Check sheet for the modelled part. Datum: model origin and axes. Units: mm. A direction names the side the tool comes from. Give positions to 0.01 mm unless a question says otherwise; leave off trailing zeros. Loops run counter-clockwise (first coordinate to the right, second up) from the corner with the lowest first, then second, coordinate; pieces in that order, holes last. Notation, with made-up numbers: (65.25, -22) -> (123.25, -22) arc R20 ccw to (123.25, 8) -> close; hole circle Ø2 at (43, -3.75). An arc over 180 degrees is marked (long way). Write each question's results on one line, items separated by ' | '. Start each with the question number.
Item 1: Scan lines: line 1 along X through (y, z) = (-4.75, 5.2); line 2 along Z through (x, y) = (3.7, -4.8); line 3 along Z through (x, y) = (15.5, 11.5). Record each from-to range of solid material in increasing order.
Item 2: Cross-section at A-A on x = 12.7. Enter the section's corners in (y, z).
Item 3: Access from +Z, -Z, +X, -X, +Y, -Y to the whole of each face (thin tool, end or side, straight path). Record for faces 4 (the face through (6, -5.427, 3)), 5 (the face through (-1.3, -4, 5)), 6 (the face through (8, -3.427, 7)).
Item 4: Cross-section at D-D on z = 0.75. Enter the section's corners in (x, y).
Item 5: Gauge pin test, flat ends, axial feed: pin 1 Ø2 at (x, z) = (12.7, 5.2) entering from +Y (1 decimal); pin 2 Ø4 at (y, z) = (1.5, 3) entering from -X; pin 3 Ø5 at (y, z) = (2.5, 2) entering from +X; pin 4 Ø5 at (x, z) = (-15, 1) entering from +Y. Record the tip position at first contact, or that the pin passes through.
Item 6: Mould release check, pull along X, two halves, no side actions. Record for faces 1 (the face through (0, 5, 2)), 2 (the face through (-18.003, -15.713, 0.986)), 3 (the face through (-12.435, -12.035, 0.986)): pulls with the +X half, pulls with the -X half, needs draft (parallel to the pull), parting line crosses it, or undercut.
Item 7: Cross-section at B-B on z = 5.2. Enter the section's corners in (x, y).
Autodesk Inventor part; units mm, degrees
ref_plane "Work Plane2" through (-1.3, -10.427, 8.7) normal (0, 0, 1) x (1, 0, 0)
ref_plane "YZ Plane" through (0, 0, 0) normal (1, 0, 0) x (0, 1, 0)
ref_plane "XZ Plane" through (0, 0, 0) normal (0, 1, 0) x (-1, 0, 0)
ref_plane "Work Plane1" through (0, 0, 0) normal (0, 0, 1) x (1, 0, 0)
sketch "Sketch2" plane through (0, 0, 0) normal (0, 0, 1) x (1, 0, 0)
  circle A0 centre (-17.6777, 17.6777) radius 3
  circle A1 centre (17.6777, 17.6777) radius 3
  circle A2 centre (-17.6777, -17.1777) radius 3
  line L0 (17.7, -5.427) -> (-1.3, -5.427)
  line L1 (-1.3, -5.427) -> (17.7, -5.427)
  line L2 (17.7, -5.427) -> (17.7, -3.927)
  line L3 (17.7, -3.927) -> (-1.3, -3.927)
  line L4 (-1.3, -3.927) -> (-1.3, -5.427)
  arc A3 (-15.9573, 20.1354) -> (15.9573, 20.1354) centre (0, 42.9323) ccw
  arc A4 (-20.3689, -15.8521) -> (-20.3689, 16.3521) centre (-53.0613, 0.25) ccw
  arc A5 (-14.9864, -18.5032) -> (-11, -5.427) centre (-53.0613, 0.25) ccw
  line L5 (-11, -5.427) -> (-1.3, -5.427)
  arc A6 (20.5658, 16.8661) -> (17.7, -3.927) centre (94.5659, -3.927) ccw
  circle A7 centre (-17.6777, 17.6777) radius 1.5
  circle A8 centre (17.6777, 17.6777) radius 1.5
  circle A9 centre (-17.6777, -17.1777) radius 1.5
  point P0 (0, 0)
  point P1 (-10.5, -5.427)
  dimension "d6" = 19
  dimension "d7" = 1.5
  dimension "d9" = 0.5
  dimension "d10" = 3
  dimension "d11" = 3
  dimension "d12" = 3
extrude "Extrusion1" add sketch "Sketch2" along normal blind 2
sketch "Sketch3" plane through (0, 0, 2) normal (0, 0, 1) x (1, 0, 0)
  line L0 (-11, -5.427) -> (17.7, -5.427)
  line L1 (17.7, -5.427) -> (-1.3, -5.427)
  line L2 (-1.3, -5.427) -> (-1.3, -3.427)
  line L3 (-1.3, -3.427) -> (17.7, -3.427)
  line L4 (17.7, -3.427) -> (17.7, -5.427)
  point P0 (0, 0)
  dimension "d15" = 19
  dimension "d16" = 2
ref_plane "Work Plane2" through (-1.3, -10.427, 8.7) normal (0, 0, 1) x (1, 0, 0)
extrude "Extrusion2" add sketch "Sketch3" along normal up to surface (6.7 mm away)
sketch "Sketch4" plane through (-1.3, -3.427, 2) normal (0, 1, 0) x (1, 0, 0)
  circle A0 centre (14, -3.2) radius 1.25
  circle A1 centre (5, -3.2) radius 1.25
  circle A2 centre (5, -3.2) radius 3
  circle A3 centre (14, -3.2) radius 3
  point P0 (1.3, 2)
  dimension "d20" = 6
  dimension "d21" = 6
fillet "Fillet1" radius 4 1 edges at (8.2, -3.427, 2)
extrude "Extrusion3" cut sketch "Sketch4" along normal blind 10 contours A0 | A1 | A2 | A3
hole "Hole1" at (3.7, -3.427, 5.2) direction (0, -1, 0) diameter 2.5 end through all
hole "Hole2" at (12.7, -3.427, 5.2) direction (0, -1, 0) diameter 2.5 end through all
properties part number "FanMount"
Answer sheet:
1) line 1: x = -1.3 to 2.45, 4.95 to 11.45, 13.95 to 17.7 | line 2: z = 0 to 3.95, 6.45 to 8.7 | line 3: z = 0 to 2
2) outline: (-5.43, 0) -> (18.17, 0) -> (18.17, 2) -> (0.57, 2) arc R4 cw to (-0.68, 2.2) -> (-3.43, 2.2) -> (-3.43, 3.95) -> (-5.43, 3.95) -> close; (-5.43, 6.45) -> (-3.43, 6.45) -> (-3.43, 8.7) -> (-5.43, 8.7) -> close
3) face 4: +Z, -Z, +X, -Y | face 5: +Z, -X, +Y, -Y | face 6: +Z, +Y
4) outline: (-20.37, -15.85) arc R3 ccw to (-14.99, -18.5) arc R42.44 ccw to (-11, -5.43) -> (17.7, -5.43) -> (17.7, -3.93) arc R76.87 cw to (20.57, 16.87) arc R3 ccw to (15.96, 20.14) arc R27.83 cw to (-15.96, 20.14) arc R3 ccw to (-20.37, 16.35) arc R36.44 cw to start; hole circle Ø3 at (-17.68, -17.18); hole circle Ø3 at (-17.68, 17.68); hole circle Ø3 at (17.68, 17.68)
5) pin 1: passes through | pin 2: stops at x = -16.74 | pin 3: stops at x = 18.22 | pin 4: stops at y = 20.67
6) face 1: needs draft | face 2: undercut | face 3: pulls with the +X half
7) outline: (-1.3, -5.43) -> (2.45, -5.43) -> (2.45, -3.43) -> (0.7, -3.43) -> (0.7, -3.35) -> (-1.3, -3.35) -> close; (4.95, -5.43) -> (11.45, -5.43) -> (11.45, -3.43) -> (9.7, -3.43) -> (9.7, -3.35) -> (6.7, -3.35) -> (6.7, -3.43) -> (4.95, -3.43) -> close; (13.95, -5.43) -> (17.7, -5.43) -> (17.7, -3.35) -> (15.7, -3.35) -> (15.7, -3.43) -> (13.95, -3.43) -> close
